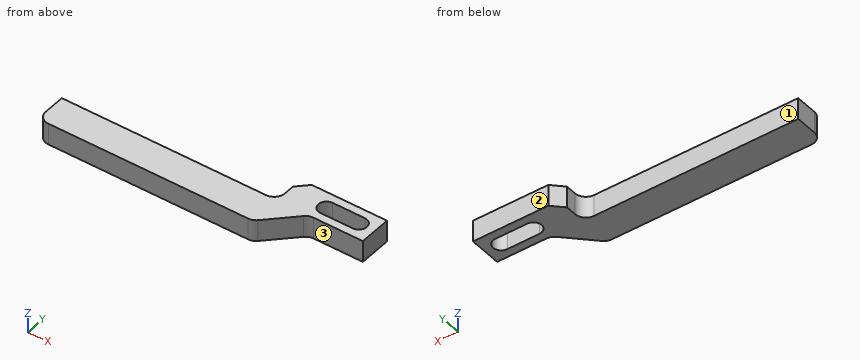
Autodesk Inventor part; units mm, degrees
ref_plane "YZ Plane" through (0, 0, 0) normal (1, 0, 0) x (0, 1, 0)
ref_plane "XZ Plane" through (0, 0, 0) normal (0, 1, 0) x (-1, 0, 0)
ref_plane "XY Plane" through (0, 0, 0) normal (0, 0, 1) x (1, 0, 0)
sketch "Sketch1" plane through (0, 0, 0) normal (0, 0, 1) x (1, 0, 0)
  line L0 (-44.45, -4.7625) -> (44.45, -4.7625)
  line L1 (44.45, -4.7625) -> (44.45, 4.7625)
  line L2 (44.45, 4.7625) -> (-44.45, 4.7625)
  line L3 (-44.45, 4.7625) -> (-44.45, -4.7625)
  line L4 (-44.45, -4.7625) -> (44.45, 4.7625) construction
  line L5 (44.45, -4.7625) -> (-44.45, 4.7625) construction
  line L6 (44.45, 4.7625) -> (19.05, 4.7625)
  line L7 (19.05, 4.7625) -> (19.05, 14.2875)
  line L8 (19.05, 14.2875) -> (44.45, 14.2875)
  line L9 (44.45, 14.2875) -> (44.45, 4.7625)
  line L10 (19.05, -4.7625) -> (28.575, 4.7625)
  line L11 (44.45, 9.525) -> (19.05, 9.525) construction
  line L12 (25.4, 14.2875) -> (25.4, 4.7625) construction
  circle A0 centre (39.6875, 9.525) radius 1.7526 construction
  circle A1 centre (30.1625, 9.525) radius 1.7526 construction
  line L13 (39.6875, 9.525) -> (30.1625, 9.525) construction
  line L14 (39.6875, 11.9063) -> (30.1625, 11.9062)
  line L15 (30.1625, 7.1437) -> (39.6875, 7.1437)
  arc A2 (39.6875, 7.1437) -> (39.6875, 11.9063) centre (39.6875, 9.525) ccw
  arc A3 (30.1625, 11.9062) -> (30.1625, 7.1437) centre (30.1625, 9.525) ccw
  point P0 (0, 0)
  point P1 (19.05, 4.7625)
  point P2 (34.925, 9.525)
  dimension "d0" = 88.9
  dimension "d1" = 9.525
  dimension "d2" = 25.4
  dimension "d3" = 9.525
  dimension "d4" = 45
  dimension "d11" = 25.4
  dimension "d18" = 19.05
  dimension "d19" = 3.5052
  dimension "d20" = 4.7625
  dimension "d21" = 3.5052
  dimension "d22" = 4.7625
  dimension "d23" = 4.7625
extrude "Extrusion1" add sketch "Sketch1" along normal blind 6.35 contours L3 L2 L10 L0 | L2 L7 L8 L9
fillet "Fillet1" radius 3.175 3 edges at (19.05, 4.7625, 3.175) (28.575, 4.7625, 3.175) (19.05, -4.7625, 3.175)
chamfer "Chamfer2" distance 3.175 angle 45 1 edges at (19.05, 14.2875, 3.175)
fillet "Fillet4" radius 3.175 1 edges at (-44.45, -4.7625, 3.175)
equation "\"d22\" = d20"
properties part number "Teeth" material "Aluminum 6061"
For this review, take the finished solid that the model builds, in its own axes (mm). Face numbers are marked on the shaded views. A direction names the side the tool comes from. Coordinates: 2 decimals unless noted, no trailing zeros. Write each loop counter-clockwise with the first axis right and the second up, starting at its lowest first coordinate (ties: lowest second). Pieces come first, ordered by that corner, then holes. Notation, with made-up numbers: (80.5, 42) - (118.5, 42) arc R23 ccw to (118.5, 81) - close; hole circle Ø4 at (49, 3). An arc over 180 degrees is marked (long way). Put each result on its own line as item: value.
1. Add section C-C, the plane x = 10. Give the boundary of the cut face in (y, z).
Values found:
outline: (-4.76, 0) - (4.76, 0) - (4.76, 6.35) - (-4.76, 6.35) - close
2. Wall thickness on probe 1 along X at (y, z) = (9.75, 2); probe 2 along Y at (x, z) = (39, 3.75); probe 3 along Y at (x, z) = (-17, 4): over which ranges is each line inside the solid? List them lowest first.
Values found:
probe 1: 19.05 to 27.79, 42.06 to 44.45
probe 2: 4.76 to 7.14, 11.91 to 14.29
probe 3: -4.76 to 4.76
3. Machinability: for the marked faces 1, 2 and 3, which of the approach directions +Z, -Z, +X, -X, +Y, -Y give a long, thin tool a straight path to every point of the face, cutting with its end or side? Answer none if there is none.
Values found:
face 1: +Z, -Z, -X, +Y
face 2: +Z, -Z, +X, -X, +Y
face 3: +Z, -Z, +X, -Y
4. Add section B-B, the plane y = 9.5. Give the boundary of the cut face in (x, z), then the cut area to 3 significant figures.
Values found:
outline: (19.05, 0) - (27.78, 0) - (27.78, 6.35) - (19.05, 6.35) - close; (42.07, 0) - (44.45, 0) - (44.45, 6.35) - (42.07, 6.35) - close
area: 70.6 mm²
5. For pin 1 (3.5 mm diameter, centred on y = 10, z = 4, fed in from -X), flat-tipped, find the tip position at first contact; note if it passes through.
Values found:
pin 1: x = 19.05
6. Add section D-D, the plane y = 5.75. Give the boundary of the cut face in (x, z), then the cut area to 3 significant figures.
Values found:
outline: (18.18, 0) - (44.45, 0) - (44.45, 6.35) - (18.18, 6.35) - close
area: 167 mm²
